The listing builds one solid part. Answer for the finished solid, in the listing's coordinates (mm). Face numbers are marked on the shaded views. A direction names the side the tool comes from. Coordinates: 2 decimals unless noted, no trailing zeros. Order: outer loops, then holes, each group sorted by start corner. A loop starts at its lowest first (then second) coordinate and runs counter-clockwise, first axis right, second up. Notation, with made-up numbers: (-2.5, 23.25) -> (21.5, 23.25) arc R23 ccw to (21.5, 56.25) -> close; hole circle Ø11 at (10.25, 35). An arc over 180 degrees is marked (long way). Answer in a Markdown table with one row per item.
```python
from build123d import *

# Parameters (mm, degrees)
BASE_FLANGE1_DEPTH    = 2
EDGE_FLANGE1_DEPTH    = 25
SKETCH19_R            = 4
CUT_EXTRUDE2_DEPTH    = 58.225619191
M3X0_5_TAPPED_HOLE1_D = 3
SKETCH22_R            = 4
CUT_EXTRUDE3_DEPTH    = 77.018231312
M3X0_5_TAPPED_HOLE2_D = 3


# Sheet-metal steps are written as plain solids
with BuildPart() as part:
    # Sketch8 → Base-Flange1 (new body)
    with BuildSketch(Plane.XY):
        with BuildLine():
            Line((-12.5, 0), (12.5, 0))
            Line((12.5, 0), (12.5, 1.008188695))
            ThreePointArc((12.5, 1.008188695), (11.396253221, 6.557098465), (8.253048327, 11.261237023))
            Line((8.253048327, 11.261237023), (-14.170526855, 33.684812205))
            ThreePointArc((-14.170526855, 33.684812205), (-30.17766953, 33.684812205), (-30.17766953, 17.67766953))
            Line((-30.17766953, 17.67766953), (-12.5, 0))
        make_face()
    extrude(amount=-BASE_FLANGE1_DEPTH)

    # Edge-Flange1 section (across the edge) → Edge-Flange1 (add)
    with BuildSketch(Plane(origin=(12.5, -2, -2), x_dir=(0, 1, 0), z_dir=(-1, 0, 0))):
        with BuildLine():
            Line((-2, 2), (-2, 26))
            Line((-2, 26), (0, 26))
            Line((0, 26), (0, 2))
            ThreePointArc((0, 2), (0.585786438, 0.585786438), (2, 0))
            Line((2, 0), (2, -2))
            ThreePointArc((2, -2), (-0.828427125, -0.828427125), (-2, 2))
        make_face()
    extrude(amount=EDGE_FLANGE1_DEPTH)

    # Sketch19 → Cut-Extrude2 (cut, through all)
    with BuildSketch(Plane.XY):
        with Locations((-22.174098192, 25.681240867)):
            Circle(SKETCH19_R)
    extrude(amount=-CUT_EXTRUDE2_DEPTH, mode=Mode.SUBTRACT)

    # M3x0.5 Tapped Hole1 (through all)
    with Locations(Plane.XY):
        with Locations((-27.123845661, 30.630988335), (-27.123845661, 20.731493399), (-17.224350724, 20.731493399), (-17.224350724, 30.630988335), (-4.072164594, 7.579307269)):
            Hole(M3X0_5_TAPPED_HOLE1_D / 2)

    # Mirror1: part across plane


with BuildPart() as part_1:
    add(part.part)
    add(part.part.mirror(Plane(origin=(12.5, -4, -28), x_dir=(1, 0, 0), z_dir=(0, 0, 1))))

    # Sketch22 → Cut-Extrude3 (cut, through all)
    with BuildSketch(Plane(origin=(0, -2, 0), x_dir=(1, 0, 0), z_dir=(0, 1, 0))):
        with Locations(Location((0, 28, 0), (0, 0, 270))):
            Circle(SKETCH22_R)
    extrude(amount=-CUT_EXTRUDE3_DEPTH, mode=Mode.SUBTRACT)

    # M3x0.5 Tapped Hole2 (through all)
    with Locations(Plane(origin=(0, -2, 0), x_dir=(1, 0, 0), z_dir=(0, 1, 0))):
        with Locations((7, 28), (-7, 28), (0, 35), (0, 21), (0, 9.4), (0, 46.6)):
            Hole(M3X0_5_TAPPED_HOLE2_D / 2)


solid = part_1.part
```
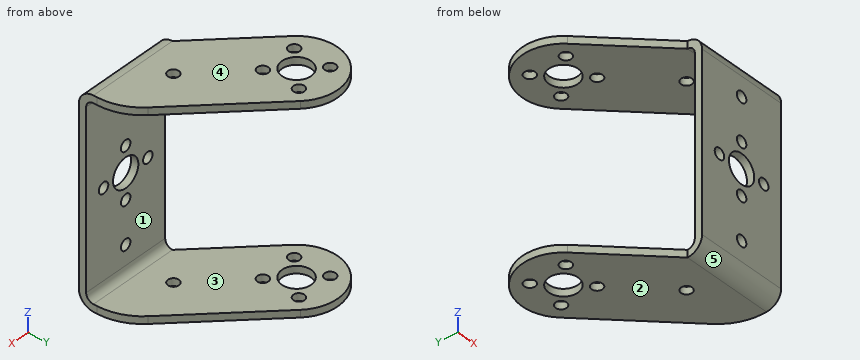
(1) A cutting plane is placed at B-B, the plane z = -28. Determine the outline of the cut face in (x, y).
Check values:
| item | result |
|---|---|
| outline | (-12.5, -4) -> (-8.5, -4) -> (-8.5, -2) -> (-12.5, -2) -> close; (-5.5, -4) -> (-4, -4) -> (-4, -2) -> (-5.5, -2) -> close; (4, -4) -> (5.5, -4) -> (5.5, -2) -> (4, -2) -> close; (8.5, -4) -> (12.5, -4) -> (12.5, -2) -> (8.5, -2) -> close |
(2) Flat-ended cylindrical pins translate along their axes: pin 1 (4 mm diameter, centred on x = -17, y = 29.5, fed in from +Z); pin 2 (4 mm diameter, centred on x = 0, z = -46.6, fed in from +Y); pin 3 (2.5 mm diameter, centred on x = -4.07, y = 7.58, fed in from +Z). Find the tip coordinate at first contact, or state that the pin passes through.
Check values:
| item | result |
|---|---|
| pin 1 | z = 0 |
| pin 2 | y = -2 |
| pin 3 | through |
(3) A cutting plane is placed at D-D, the plane x = 0. Count the separate pieces of the cut face and the enclosed holes in it, then the cut area to 3 significant figures.
Check values:
| item | result |
|---|---|
| separate pieces | 6 |
| enclosed holes | 0 |
| area | 153 mm² |
(4) For a pull along Z with two mould halves and no side action, classify the marked faces 3, 4 and 5 as released by +Z, released by -Z, zero draft, split by the parting line, or undercut.
Check values:
| item | result |
|---|---|
| face 3 | undercut |
| face 4 | released by +Z |
| face 5 | released by -Z |
(5) A cutting plane is placed at C-C, the plane x = 7. Determine the outline of the cut face in (y, z), then the cut area to 3 significant figures.
Check values:
| item | result |
|---|---|
| outline | (-4, -52) arc R4 ccw to (0, -56) -> (12.51, -56) -> (12.51, -54) -> (0, -54) arc R2 cw to (-2, -52) -> (-2, -29.5) -> (-4, -29.5) -> close; (-4, -26.5) -> (-2, -26.5) -> (-2, -4) arc R2 cw to (0, -2) -> (12.51, -2) -> (12.51, 0) -> (0, 0) arc R4 ccw to (-4, -4) -> close |
| area | 159 mm² |
(6) A cutting plane is placed at A-A, the plane z = -9.4. Determine the outline of the cut face in (x, y), then the cut area to 3 significant figures.
Check values:
| item | result |
|---|---|
| outline | (-12.5, -4) -> (-1.5, -4) -> (-1.5, -2) -> (-12.5, -2) -> close; (1.5, -4) -> (12.5, -4) -> (12.5, -2) -> (1.5, -2) -> close |
| area | 44.0 mm² |
(7) Which of the six approach directions +Z, -Z, +X, -X, +Y, -Y give full straight-line access (tool end or side, diameter ignored) to the marked faces 1 and 2?
Check values:
| item | result |
|---|---|
| face 1 | +X, -X, +Y |
| face 2 | -Z, +X, -X, +Y, -Y |
(8) Find the intervals of material crossed by line 1 along X through (y, z) = (-3, -28); line 2 along Z through (x, y) = (-5, 5); line 3 along Y through (x, z) = (10.5, -23), in increasing order. Write a range as from..to.
Check values:
| item | result |
|---|---|
| line 1 | -12.5..-8.5, -5.5..-4, 4..5.5, 8.5..12.5 |
| line 2 | -56..-54, -2..0 |
| line 3 | -4..-2 |
